from build123d import *

# Parameters (mm, degrees)
F0_R     = 4.987569
F1_DEPTH = 20
F2_DEPTH = 50


with BuildPart() as f1:
    # F0 (on Right) → F1 (new body)
    with BuildSketch(Plane.YZ):
        with BuildLine():
            ThreePointArc((-20, -420), (-18.535534, -423.535534), (-15, -425))
            Line((-15, -425), (15, -425))
            ThreePointArc((15, -425), (18.535534, -423.535534), (20, -420))
            Line((20, -420), (20, 405))
            ThreePointArc((20, 405), (14.142136, 419.142136), (0, 425))
            ThreePointArc((0, 425), (-14.142136, 419.142136), (-20, 405))
            Line((-20, 405), (-20, -420))
        make_face()
        with Locations((0, 405)):
            Circle(F0_R, mode=Mode.SUBTRACT)
    extrude(amount=F1_DEPTH)

    # F0 (on Right) → F2 (join)
    with BuildSketch(Plane.YZ):
        with Locations((0, 405)):
            Circle(F0_R)
    extrude(amount=F2_DEPTH)


solid = f1.part
Design review of the part built by this model. Coordinates are the model's own, in mm. Coordinates: 2 decimals unless noted, no trailing zeros. Loops run counter-clockwise (first coordinate to the right, second up) from the corner with the lowest first, then second, coordinate; pieces in that order, holes last. Notation, with made-up numbers: (45.5, -39.5) -> (59.5, -39.5) arc R15 ccw to (59.5, -28.5) -> close; hole circle Ø8 at (67.5, 0). An arc over 180 degrees is marked (long way). Use a Markdown table: item, result. Add a question column.
Item 1: We need section A-A, the plane z = -174. Write out the cut boundary in (x, y).
Item 2: Wall thickness on L1, parallel to X at y = -1, z = 15; L2, parallel to Z at x = 18, y = -2; L3, parallel to Z at x = 20.5, y = -2: over which ranges is each line inside the solid? List them lowest first. Write a range as from..to.
Item 3: We need section B-B, the plane x = 38.5. Write out the cut boundary in (y, z), and give its area (4 significant figures).
Item 4: Clearance check with flat-ended pins moving along their axes: P1, Ø20, axis at y = 9.5, z = 33, coming from the +X side; P2, Ø1, axis at y = -0.5, z = -269.5, coming from the -X side; P3, Ø10, axis at x = 19.5, y = -6.5, coming from the +Z side; P4, Ø12, axis at x = 23, y = -9, coming from the +Z side. State where each tip first meets the part, or that it passes through.
Numbers:
| question | item | result |
|---|---|---|
| 1 | outline | (0, -20) -> (20, -20) -> (20, 20) -> (0, 20) -> close |
| 2 | L1 | x = 0..20 |
| 2 | L2 | z = -425..424.9 |
| 2 | L3 | z = 400.43..409.57 |
| 3 | outline | circle Ø9.98 at (0, 405) |
| 3 | area | 78.15 mm^2 |
| 4 | P1 | stops at x = 20 |
| 4 | P2 | stops at x = 0 |
| 4 | P3 | stops at z = 424.94 |
| 4 | P4 | stops at z = 424.63 |
